from build123d import *

# Parameters (mm, degrees)
SKETCH1_W                        = 25.4
SKETCH1_H                        = 101.6
SKETCH1_W_2                      = 19.05
SKETCH1_H_2                      = 95.25
EXTRUDE_THIN1_DEPTH              = 240.875
SKETCH2_W                        = 31.75
SKETCH2_H                        = 101.6
CUT_EXTRUDE1_DEPTH               = 22.86
SKETCH3_W                        = 35.71875
SKETCH3_H                        = 6.35
CUT_EXTRUDE2_DEPTH               = 26.4
F_10_CLEARANCE_HOLE1_D           = 4.9784
MIRROR2_COPY_1_D                 = 4.9784
FILLET1_R                        = 3.175
SKETCH7_R                        = 6.223
CUT_EXTRUDE3_DEPTH               = 3.175
F_1_4_CLEARANCE_HOLE1_AT_2_COUNT = 2
F_1_4_CLEARANCE_HOLE1_AT_2_PITCH = 60.325


with BuildPart() as part:
    # Sketch1 → Extrude-Thin1 (new body, symmetric)
    with BuildSketch(Plane.XY):
        Rectangle(SKETCH1_W, SKETCH1_H)
        Rectangle(SKETCH1_W_2, SKETCH1_H_2, mode=Mode.SUBTRACT)
    extrude(amount=EXTRUDE_THIN1_DEPTH, both=True)

    # Sketch2 → Cut-Extrude1 (cut)
    with BuildSketch(Plane.ZY.offset(12.7)):
        with Locations((225, 0)):
            Rectangle(SKETCH2_W, SKETCH2_H)
    cut_extrude1 = extrude(amount=-CUT_EXTRUDE1_DEPTH, mode=Mode.SUBTRACT)

    # Sketch3 → Cut-Extrude2 (cut, through all)
    with BuildSketch(Plane.ZY.offset(12.7)):
        with Locations((223.015625, -47.625)):
            Rectangle(SKETCH3_W, SKETCH3_H)
    cut_extrude2 = extrude(amount=-CUT_EXTRUDE2_DEPTH, mode=Mode.SUBTRACT)

    # #10 Clearance Hole1 (through all)
    with Locations(Plane.ZY.offset(-10.16)):
        with Locations((225, 33.02)):
            f_10_clearance_hole1 = Hole(F_10_CLEARANCE_HOLE1_D / 2)

    # Mirror1: #10 Clearance Hole1 across plane
    add(f_10_clearance_hole1.mirror(Plane.ZX), mode=Mode.SUBTRACT)

    # Mirror2: Cut-Extrude1, Cut-Extrude2, #10 Clearance Hole1 across plane
    add(cut_extrude1.mirror(Plane.XY), mode=Mode.SUBTRACT)
    add(cut_extrude2.mirror(Plane.XY), mode=Mode.SUBTRACT)
    add(f_10_clearance_hole1.mirror(Plane.XY), mode=Mode.SUBTRACT)

    # Mirror2 copy 1 (through all)
    with Locations(Plane(origin=(10.16, 0, 0), x_dir=(0, 0, -1), z_dir=(-1, 0, 0))):
        with Locations((225, 33.02)):
            Hole(MIRROR2_COPY_1_D / 2)

    # Fillet1
    fillet1_edges = [part.edges().sort_by_distance(p)[0] for p in [
        (11.1125, -44.45, 205.15625),
        (-11.1125, -44.45, 205.15625),
        (-11.1125, -44.45, -205.15625),
        (11.1125, -44.45, -205.15625),
    ]]
    fillet(fillet1_edges, radius=FILLET1_R)

    # Sketch7 → Cut-Extrude3 (cut)
    with BuildSketch(Plane.ZY.offset(-9.525)):
        with Locations(Location((182.1375, -41.275, 0), (0, 0, 270))):  # turned: the seam where the file's is
            Circle(SKETCH7_R)
        with Locations(Location((182.1375, 19.05, 0), (0, 0, 270))):  # turned: the seam where the file's is
            Circle(SKETCH7_R)
    cut_extrude3 = extrude(amount=-CUT_EXTRUDE3_DEPTH, mode=Mode.SUBTRACT)

    # Sketch8 → 1/4 Clearance Hole1 (revolve, cut)
    with BuildSketch(Plane(origin=(-12.7, 19.05, 182.1375), x_dir=(0, 0, 1), z_dir=(0, 1, 0))):
        Polygon((0, 0), (0, 3.175), (3.8989, 3.175), (3.2639, 2.54), (3.2639, 0.635), (3.8989, 0), align=None)
    f_1_4_clearance_hole1 = revolve(axis=Axis((-19.05, 19.05, 182.1375), (1, 0, 0)), mode=Mode.SUBTRACT)

    # 1/4 Clearance Hole1 at 2: 1/4 Clearance Hole1 ×2
    with Locations(*[(0, -i * F_1_4_CLEARANCE_HOLE1_AT_2_PITCH, 0) for i in range(1, F_1_4_CLEARANCE_HOLE1_AT_2_COUNT)]):
        add(f_1_4_clearance_hole1, mode=Mode.SUBTRACT)

    # Mirror3: Cut-Extrude3, 1/4 Clearance Hole1 across plane
    add(cut_extrude3.mirror(Plane.XY), mode=Mode.SUBTRACT)
    add(f_1_4_clearance_hole1.mirror(Plane.XY), mode=Mode.SUBTRACT)

    # Mirror3 copy 1 sketch → Mirror3 copy 1 (revolve, cut)
    with BuildSketch(Plane(origin=(-12.7, -41.275, -182.1375), x_dir=(0, 0, -1), z_dir=(0, 1, 0))):
        Polygon((0, 0), (0, -3.175), (3.8989, -3.175), (3.2639, -2.54), (3.2639, -0.635), (3.8989, 0), align=None)
    revolve(axis=Axis((-19.05, -41.275, -182.1375), (-1, 0, 0)), mode=Mode.SUBTRACT)


solid = part.part
Work out the finished part from the listing and answer in its coordinate system (mm). A direction names the side the tool comes from. Coordinates: 2 decimals unless noted, no trailing zeros. Write each loop counter-clockwise with the first axis right and the second up, starting at its lowest first coordinate (ties: lowest second). Pieces come first, ordered by that corner, then holes. Notation, with made-up numbers: M 79.5,21 L 91.5,21 A14 cw 91.5,40 Z; hole C 40,23.25 d9. An arc over 180 degrees is marked long. Answer as CSV lines item,"result". Start each with the question number.
Item 1: Section B-B on x = 1 is taken. Write down the section's boundary in (y, z) (3 decimals).
Item 2: A tool of negligible diameter and unlimited length cuts with its end or side. For faces 1 (the face through (11.09, 19.86, -188.308)), 2 (the face through (-10, 6, 209.125)), 3 (the face through (0, -50.8, 3)), 4 (the face through (10.16, 4, -225)), 5 (the face through (-9.525, -1, 3)), from which of +Z, -Z, +X, -X, +Y, -Y can it reach the whole face along a straight path? Write none if from no direction.
Item 3: Flat-ended cylindrical pins translate along their axes: P1, Ø7.5, axis at y = -41.28, z = -182.14, coming from the +X side; P2, Ø6.5, axis at y = 33.02, z = -225, coming from the -X side; P3, Ø8.5, axis at y = 19.05, z = 182.14, coming from the +X side (3 decimals). Find the tip coordinate at first contact, or state that the pin passes through.
Item 4: Determine the mould class of faces 6 (the face through (10.16, 4, 225)), 7 (the face through (11.09, -40.465, 188.308)), 8 (the face through (0, 50.8, 3)), 9 (the face through (0, 47.625, 3)) for opening direction Y: released by +Y, released by -Y, zero draft, split by the parting line, or undercut.
Item 5: Section A-A on y = -7 is taken. Write down the section's boundary in (x, z) (3 decimals), and give its area (3 significant figures).
Item 6: Consider L1, parallel to Y at x = 11.05, z = 225; L2, parallel to X at y = -32, z = -45.5 (3 decimals); L3, parallel to Y at x = -7.5, z = -69 (3 decimals). Determine where each line is inside the solid, lowest interval first.
Item 7: Section C-C on z = -31 is taken. Write down the section's boundary in (x, y) (3 decimals).
Checks:
1,outline,"M -50.8,-205.156 L -47.625,-205.156 L -47.625,205.156 L -50.8,205.156 Z; M 47.625,-209.125 L 50.8,-209.125 L 50.8,209.125 L 47.625,209.125 Z"
2,face 1,"+X"
2,face 2,"+Z, -X, +Y, -Y"
2,face 3,"+Z, -Z, +X, -X, -Y"
2,face 4,"-Z, -X, +Y, -Y"
2,face 5,"+Z, -Z"
3,P1,"stops at x = -9.67"
3,P2,"stops at x = 10.16"
3,P3,"stops at x = -9.525"
4,face 6,"zero draft"
4,face 7,"undercut"
4,face 8,"released by +Y"
4,face 9,"undercut"
5,outline,"M -12.7,-209.125 L -9.525,-209.125 L -9.525,209.125 L -12.7,209.125 Z; M 9.525,-209.125 L 10.16,-209.125 L 10.16,-240.875 L 12.7,-240.875 L 12.7,240.875 L 10.16,240.875 L 10.16,209.125 L 9.525,209.125 Z"
5,area,"2,820 mm²"
6,L1,"y = -44.45 to -35.51, -30.53 to 30.53, 35.51 to 50.8"
6,L2,"x = -12.7 to -9.525, 9.525 to 12.7"
6,L3,"y = -50.8 to -47.625, 47.625 to 50.8"
7,outline,"M -12.7,-50.8 L 12.7,-50.8 L 12.7,50.8 L -12.7,50.8 Z; hole M -9.525,-47.625 L 9.525,-47.625 L 9.525,47.625 L -9.525,47.625 Z"
